Work out the finished part from the listing and answer in its coordinate system (mm). A direction names the side the tool comes from. Round coordinates to 2 decimals unless told otherwise and drop trailing zeros. Loops run counter-clockwise (first coordinate to the right, second up) from the corner with the lowest first, then second, coordinate; pieces in that order, holes last.
from build123d import *

# Parameters (mm, degrees)
SKETCH1_R           = 2.95
SKETCH1_R_2         = 2.25
BOSS_EXTRUDE1_DEPTH = 1.9
SKETCH2_R           = 0.875
SKETCH2_R_2         = 0.5
BOSS_EXTRUDE2_DEPTH = 1.5
SKETCH3_R           = 2.875
SKETCH3_R_2         = 2.125
BOSS_EXTRUDE3_DEPTH = 0.5
CUT_EXTRUDE1_START  = -10
CUT_EXTRUDE1_DEPTH  = 10


with BuildPart() as part:
    # Sketch1 → Boss-Extrude1 (new body)
    with BuildSketch(Plane.XY):
        with Locations(Location((0, 0, 0), (0, 0, 180))):
            Circle(SKETCH1_R)
        with Locations(Location((0, 0, 0), (0, 0, 180))):
            Circle(SKETCH1_R_2, mode=Mode.SUBTRACT)
    extrude(amount=BOSS_EXTRUDE1_DEPTH)

    # Sketch2 → Boss-Extrude2 (add)
    with BuildSketch(Plane.XY.offset(1.9)):
        with BuildLine():
            Line((15.062313393, 2.247195074), (0, 3))
            Line((0, 3), (-15.062313393, 2.247195074))
            ThreePointArc((-15.062313393, 2.247195074), (-17.2, 0), (-15.062313393, -2.247195074))
            Line((-15.062313393, -2.247195074), (0, -3))
            Line((0, -3), (15.062313393, -2.247195074))
            ThreePointArc((15.062313393, -2.247195074), (17.2, 0), (15.062313393, 2.247195074))
        make_face()
        Circle(SKETCH2_R, mode=Mode.SUBTRACT)
        with Locations((6.8, 0)):
            Circle(SKETCH2_R_2, mode=Mode.SUBTRACT)
        with Locations((9.55, 0)):
            Circle(SKETCH2_R_2, mode=Mode.SUBTRACT)
        with Locations((11.95, 0)):
            Circle(SKETCH2_R_2, mode=Mode.SUBTRACT)
        with Locations((14.35, 0)):
            Circle(SKETCH2_R_2, mode=Mode.SUBTRACT)
        with Locations(Location((-14.35, 0, 0), (0, 0, 180))):
            Circle(SKETCH2_R_2, mode=Mode.SUBTRACT)
        with Locations(Location((-11.95, 0, 0), (0, 0, 180))):
            Circle(SKETCH2_R_2, mode=Mode.SUBTRACT)
        with Locations(Location((-9.55, 0, 0), (0, 0, 180))):
            Circle(SKETCH2_R_2, mode=Mode.SUBTRACT)
        with Locations(Location((-6.8, 0, 0), (0, 0, 180))):
            Circle(SKETCH2_R_2, mode=Mode.SUBTRACT)
    extrude(amount=BOSS_EXTRUDE2_DEPTH)

    # Sketch3 → Boss-Extrude3 (add)
    with BuildSketch(Plane.XY.offset(3.4)):
        Circle(SKETCH3_R)
        Circle(SKETCH3_R_2, mode=Mode.SUBTRACT)
    extrude(amount=BOSS_EXTRUDE3_DEPTH)

    # Sketch4 → Cut-Extrude1 (cut)
    with BuildSketch(Plane.XY.offset(3.4).offset(CUT_EXTRUDE1_START)):
        with BuildLine():
            Line((3.5, 2.825072207), (3.5, -2.825072207))
            Line((3.5, -2.825072207), (15.062313393, -2.247195074))
            ThreePointArc((15.062313393, -2.247195074), (17.2, 0), (15.062313393, 2.247195074))
            Line((15.062313393, 2.247195074), (3.5, 2.825072207))
        make_face()
    extrude(amount=CUT_EXTRUDE1_DEPTH, mode=Mode.SUBTRACT)


solid = part.part
Item 1: Determine the mould class of faces 4 (the face through (-7.64, -2.62, 2.64)), 5 (the face through (-7, -1, 3.4)), 6 (the face through (1.77, 2.91, 2.64)), 7 (the face through (-10.012, 0.192, 2.64)) for opening direction Y: pulls with the +Y half, pulls with the -Y half, needs draft (parallel to the pull), parting line crosses it, or undercut.
Item 2: For faces 1 (the face through (3.5, 0, 3)), 2 (the face through (2.947, -0.13, 0.937)), 3 (the face through (-0.37, 2.85, 3.65)), determine the directions among +Z, -Z, +X, -X, +Y, -Y from which every point of the face is accessible in a straight line to the end or side of a thin tool.
Item 3: Section D-D, the plane y = 0 is taken. State how many separate pieces and enclosed holes the cut face has, plus the area to 3 significant figures.
Item 4: Section B-B, the plane y = 1.8 is taken. Give the vertices of the cut face in (x, z), plus the area to 3 significant figures.
Item 5: Section A-A, the plane x = -14.35 is taken. Give the vertices of the cut face in (y, z), plus the area to 3 significant figures.
Item 6: Each of these flat-tipped pins is pushed along its axis until it touches: P1, Ø1.8, axis at x = -8, y = -1, coming from the +Z side; P2, Ø1, axis at x = 0, y = -0.5, coming from the -Z side; P3, Ø2, axis at y = 2, z = 2, coming from the -X side. Where does it stop, or does it pass through?
Item 7: Straight lines are drawn through the part: line 1 (X direction, y = 0.05, z = 2.1); line 2 (Y direction, x = 0, z = 3.8) (3 decimals); line 3 (X direction, y = 0.75, z = 1.8). For each, find the intervals that lie inside material, in ascending order.
Item 8: Section C-C, the plane x = -11.75 is taken. Give the vertices of the cut face in (y, z).
Answer below:
1. face 4: pulls with the -Y half
1. face 5: needs draft
1. face 6: pulls with the +Y half
1. face 7: undercut
2. face 1: +Z, -Z, +X, +Y, -Y
2. face 2: -Z
2. face 3: +Z
3. separate pieces: 6
3. enclosed holes: 0
3. area: 25.8 mm2
4. outline: (-16.3, 1.9) - (-2.34, 1.9) - (-2.34, 0) - (-1.35, 0) - (-1.35, 1.9) - (1.35, 1.9) - (1.35, 0) - (2.34, 0) - (2.34, 1.9) - (3.5, 1.9) - (3.5, 3.4) - (2.24, 3.4) - (2.24, 3.9) - (1.13, 3.9) - (1.13, 3.4) - (-1.13, 3.4) - (-1.13, 3.9) - (-2.24, 3.9) - (-2.24, 3.4) - (-16.3, 3.4) - close
4. area: 34.6 mm2
5. outline: (-2.28, 1.9) - (-0.5, 1.9) - (-0.5, 3.4) - (-2.28, 3.4) - close; (0.5, 1.9) - (2.28, 1.9) - (2.28, 3.4) - (0.5, 3.4) - close
5. area: 5.35 mm2
6. P1: stops at z = 3.4
6. P2: stops at z = 1.9
6. P3: stops at x = -16.97
7. line 1: x = -17.2 to -14.85, -13.85 to -12.45, -11.45 to -10.05, -9.05 to -7.3, -6.3 to -0.87, 0.87 to 3.5
7. line 2: y = -2.875 to -2.125, 2.125 to 2.875
7. line 3: x = -2.85 to -2.12, 2.12 to 2.85
8. outline: (-2.41, 1.9) - (-0.46, 1.9) - (-0.46, 3.4) - (-2.41, 3.4) - close; (0.46, 1.9) - (2.41, 1.9) - (2.41, 3.4) - (0.46, 3.4) - close
